Build history of the part. All positions in model axes, mm. A direction names the side the tool comes from. Round coordinates to 2 decimals unless told otherwise and drop trailing zeros. Write each loop counter-clockwise with the first axis right and the second up, starting at its lowest first coordinate (ties: lowest second). Pieces come first, ordered by that corner, then holes.
1) Which spindle directions (+Z, -Z, +X, -X, +Y, -Y) get a long thin tool onto all of the face, cutting with end or side? Do faces 1 (the cylindrical face through (3.4, 7.5, 18.5)), 2 (the flat face through (3, 7.5, 13)), 3 (the flat face through (7, 4, 12)), 4 (the cylindrical face through (3.6, 7.5, 1.5)), 5 (the flat face through (3, 4, 13.5)). Say none if no direction does.
2) Saw through at B-B (z = 19.75). Write the cut outline in (x, y), plus the area to 3 significant figures.
3) Pull direction X, two halves, no side cores. Call faces 6 (the flat face through (0, 4, 12)), 7 (the cylindrical face through (4.077, 2.391, 18.57)), 8 (the flat face through (2, 4, 23.5)): +X half, -X half, draft (parallel to the pull), parting line (faces both ways), or undercut.
4) Flat gauge pins, fed straight in: pin 1 (1.5 mm diameter, centred on x = 3.5, y = 3.5, fed in from +Z); pin 2 (3 mm diameter, centred on x = 2.5, z = 20.5, fed in from -Y). Where does each tip first touch, or does it go through?
5) Saw through at A-A (y = 3.5). Write the cut outline in (x, z).
6) Wall check: probe 1 along Z at (x, y) = (3.5, 6); probe 2 along Z at (x, y) = (3.5, 3); probe 3 along Y at (x, z) = (5.75, 10.75). Give the ranges that are in metal, low to high.
7) Saw through at C-C (x = 2.5). Write the cut outline in (y, z).
8) Saw through at D-D (z = 11.75). Write the cut outline in (x, y), plus the area to 3 significant figures.
from build123d import *

# Parameters (mm, degrees)
ESQUISSE1_W             = 7
ESQUISSE1_H             = 7
BASE_EXTRUSION_DEPTH    = 23.5
BOSS_EXTRU_1_DEPTH      = 1
ESQUISSE3_R             = 1.25
ENL_V_MAT_EXTRU_1_DEPTH = 9
ENL_V_MAT_EXTRU_2_DEPTH = 0.5
ESQUISSE5_R             = 1.25
ENL_V_MAT_EXTRU_3_DEPTH = 10


with BuildPart() as part:
    # Esquisse1 → Base-Extrusion (new body)
    with BuildSketch(Plane.XY):
        with Locations((3.5, 3.5)):
            Rectangle(ESQUISSE1_W, ESQUISSE1_H)
    extrude(amount=BASE_EXTRUSION_DEPTH)

    # Esquisse2 → Boss.-Extru.1 (add)
    with BuildSketch(Plane(origin=(0, 7, 0), x_dir=(-1, 0, 0), z_dir=(0, 1, 0))):
        with BuildLine():
            Line((0, 5), (0, 15))
            ThreePointArc((0, 15), (-3.5, 18.5), (-7, 15))
            Line((-7, 15), (-7, 5))
            ThreePointArc((-7, 5), (-3.5, 1.5), (0, 5))
        make_face()
    extrude(amount=BOSS_EXTRU_1_DEPTH)

    # Esquisse3 → Enlèv. mat.-Extru.1 (cut, through all)
    with BuildSketch(Plane(origin=(0, 8, 0), x_dir=(-1, 0, 0), z_dir=(0, 1, 0))):
        with Locations((-3.5, 5)):
            Circle(ESQUISSE3_R)
    extrude(amount=-ENL_V_MAT_EXTRU_1_DEPTH, mode=Mode.SUBTRACT)

    # Esquisse4 → Enlèv. mat.-Extru.2 (cut)
    with BuildSketch(Plane(origin=(0, 8, 0), x_dir=(-1, 0, 0), z_dir=(0, 1, 0))):
        with BuildLine():
            Line((-1, 15), (-1, 7.449489743))
            ThreePointArc((-1, 7.449489743), (-3.5, 8.5), (-6, 7.449489743))
            Line((-6, 7.449489743), (-6, 15))
            ThreePointArc((-6, 15), (-3.5, 17.5), (-1, 15))
        make_face()
    extrude(amount=-ENL_V_MAT_EXTRU_2_DEPTH, mode=Mode.SUBTRACT)

    # Esquisse5 → Enlèv. mat.-Extru.3 (cut)
    with BuildSketch(Plane.XY.offset(23.5)):
        with Locations((3.5, 3.5)):
            Circle(ESQUISSE5_R)
    extrude(amount=-ENL_V_MAT_EXTRU_3_DEPTH, mode=Mode.SUBTRACT)


solid = part.part
Evaluation:
1. face 1: +Z, +Y
1. face 2: +Y
1. face 3: +Z, -Z, +X, +Y, -Y
1. face 4: -Z, +Y
1. face 5: +Z
2. outline: (0, 0) - (7, 0) - (7, 7) - (0, 7) - close; hole circle Ø2.5 at (3.5, 3.5)
2. area: 44.1 mm2
3. face 6: -X half
3. face 7: undercut
3. face 8: draft
4. pin 1: stops at z = 13.5
4. pin 2: stops at y = 0
5. outline: (0, 0) - (7, 0) - (7, 23.5) - (4.75, 23.5) - (4.75, 13.5) - (2.25, 13.5) - (2.25, 23.5) - (0, 23.5) - close; hole circle Ø2.5 at (3.5, 5)
6. probe 1: z = 0 to 3.75, 6.25 to 23.5
6. probe 2: z = 0 to 3.75, 6.25 to 13.5
6. probe 3: y = 0 to 7.5
7. outline: (0, 0) - (7, 0) - (7, 1.65) - (8, 1.65) - (8, 4.25) - (0, 4.25) - close; (0, 5.75) - (8, 5.75) - (8, 8.35) - (7.5, 8.35) - (7.5, 17.29) - (8, 17.29) - (8, 18.35) - (7, 18.35) - (7, 23.5) - (4.25, 23.5) - (4.25, 13.5) - (2.75, 13.5) - (2.75, 23.5) - (0, 23.5) - close
8. outline: (0, 0) - (7, 0) - (7, 8) - (6, 8) - (6, 7.5) - (1, 7.5) - (1, 8) - (0, 8) - close
8. area: 53.5 mm2
